Part print with two shaded views. Sizes in mm from the minimum x, y, z corner. Give positions to 0.01 mm unless a question says otherwise; leave off trailing zeros. Write each loop counter-clockwise with the first axis right and the second up, starting at its lowest first coordinate (ties: lowest second). Pieces come first, ordered by that corner, then holes. Notation, with made-up numbers: (-8.5, -23.5) - (15.5, -23.5) arc R22 ccw to (15.5, -5.5) - close; hole circle Ø9 at (13.5, -15). An arc over 180 degrees is marked (long way). One line per item, written item: value. Start each with the question number.
(1) Drop a flat-ended pin along its axis: P1, Ø5.5, axis at x = 190, y = 131, coming from the +Z side. Give the stop position or say it passes through.
(2) Mould opens along Y. For the marked faces 1 and 2 say: pulls with the +Y half, pulls with the -Y half, needs draft (parallel to the pull), parting line crosses it, or undercut.
(3) Cut at D-D, the plane z = 1. List the corners of the cut face in (x, y) (3 decimals), and give its area (3 significant figures).
(4) Cut at A-A, the plane x = 49.5. List the corners of the cut face in (y, z), and give its area (3 significant figures).
(5) Cut at B-B, the plane y = 5. List the corners of the cut face in (x, z) (3 decimals).
(6) Cut at C-C, the plane x = 190. List the corners of the cut face in (y, z) (3 decimals), and give its area (3 significant figures).
(7) Probe L1, parallel to Y at x = 190, z = 1.4 (3 decimals); L2, parallel to Y at x = 97.5, z = 1.8 (3 decimals); L3, parallel to X at y = 131, z = 2.95 (3 decimals). List the from-to ranges inside material, lowest first.
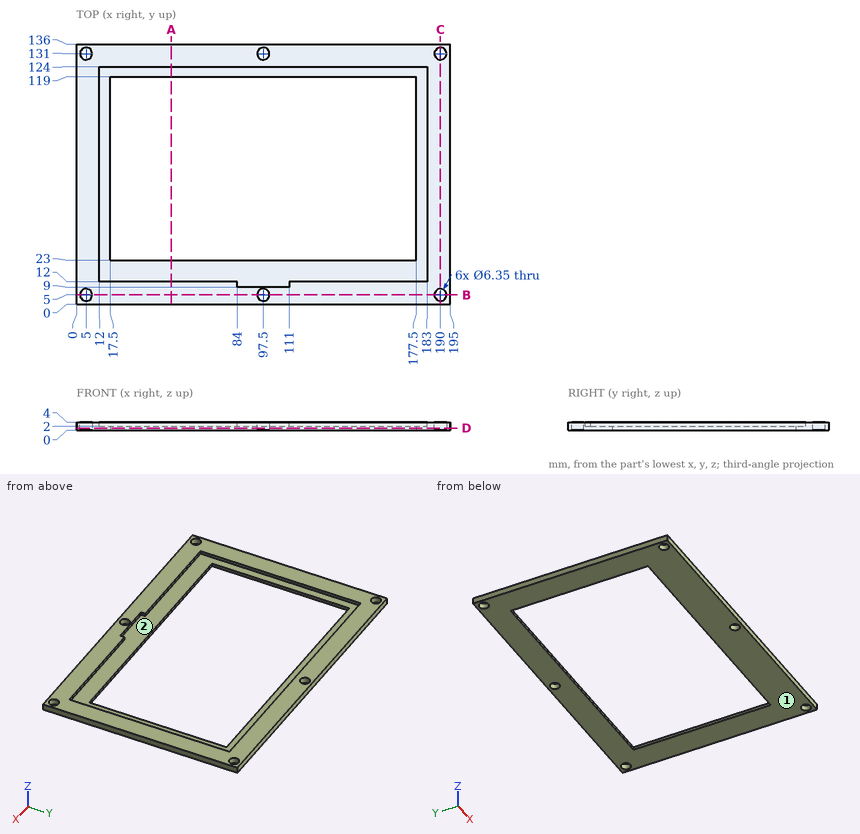
Answers follow:
1. P1: passes through
2. face 1: needs draft
2. face 2: undercut
3. outline: (0, 0) - (195, 0) - (195, 136) - (0, 136) - close; hole circle Ø6.35 at (5, 5); hole circle Ø6.35 at (5, 131); hole (17.5, 23) - (177.5, 23) - (177.5, 119) - (17.5, 119) - close; hole circle Ø6.35 at (97.5, 5); hole circle Ø6.35 at (97.5, 131); hole circle Ø6.35 at (190, 5); hole circle Ø6.35 at (190, 131)
3. area: 11,000 mm²
4. outline: (0, 0) - (23, 0) - (23, 2) - (12, 2) - (12, 4) - (0, 4) - close; (119, 0) - (136, 0) - (136, 4) - (124, 4) - (124, 2) - (119, 2) - close
4. area: 128 mm²
5. outline: (0, 0) - (1.825, 0) - (1.825, 4) - (0, 4) - close; (8.175, 0) - (94.325, 0) - (94.325, 4) - (8.175, 4) - close; (100.675, 0) - (186.825, 0) - (186.825, 4) - (100.675, 4) - close; (193.175, 0) - (195, 0) - (195, 4) - (193.175, 4) - close
6. outline: (0, 0) - (1.825, 0) - (1.825, 4) - (0, 4) - close; (8.175, 0) - (127.825, 0) - (127.825, 4) - (8.175, 4) - close; (134.175, 0) - (136, 0) - (136, 4) - (134.175, 4) - close
6. area: 493 mm²
7. L1: y = 0 to 1.825, 8.175 to 127.825, 134.175 to 136
7. L2: y = 0 to 1.825, 8.175 to 23, 119 to 127.825, 134.175 to 136
7. L3: x = 0 to 1.825, 8.175 to 94.325, 100.675 to 186.825, 193.175 to 195
